```python
from build123d import *

# Parameters (mm, degrees)
F1_DEPTH = 144
F2_W     = 86
F2_H     = 4
F2_W_2   = 4
F2_H_2   = 25
F3_DEPTH = 15
F4_W     = 54.916096
F4_H     = 4
F4_W_2   = 4
F4_H_2   = 25
F5_DEPTH = 15


with BuildPart() as f1:
    # F0 (on Front) → F1 (new body)
    with BuildSketch(Plane.XZ):
        with BuildLine():
            Line((0, 37), (0, 2))
            ThreePointArc((0, 2), (0.585786, 0.585786), (2, 0))
            Line((2, 0), (6, 0))
            ThreePointArc((6, 0), (7.414214, 0.585786), (8, 2))
            Line((8, 2), (8, 32.406905))
            Line((8, 32.406905), (20.7, 32.406905))
            Line((20.7, 32.406905), (20.7, 2))
            ThreePointArc((20.7, 2), (21.285786, 0.585786), (22.7, 0))
            Line((22.7, 0), (26.7, 0))
            ThreePointArc((26.7, 0), (28.114214, 0.585786), (28.7, 2))
            Line((28.7, 2), (28.7, 32.406905))
            Line((28.7, 32.406905), (98.7, 32.406905))
            Line((98.7, 32.406905), (98.7, 33.406905))
            Line((98.7, 33.406905), (97.45, 33.406905))
            Line((97.45, 33.406905), (97.45, 34.806905))
            Line((97.45, 34.806905), (106.75, 34.806905))
            Line((106.75, 34.806905), (106.75, 33.406905))
            Line((106.75, 33.406905), (105, 33.406905))
            Line((105, 33.406905), (105, 32.406905))
            Line((105, 32.406905), (115, 32.406905))
            Line((115, 32.406905), (120, 32.406905))
            Line((120, 32.406905), (120, 38))
            ThreePointArc((120, 38), (119.414214, 39.414214), (118, 40))
            Line((118, 40), (3, 40))
            ThreePointArc((3, 40), (0.87868, 39.12132), (0, 37))
        make_face()
        with BuildLine():
            Line((120, 24.406905), (120, 32.406905))
            Line((120, 32.406905), (115, 32.406905))
            Line((115, 32.406905), (115, 24.406905))
            ThreePointArc((115, 24.406905), (115.585786, 22.992692), (117, 22.406905))
            Line((117, 22.406905), (118, 22.406905))
            ThreePointArc((118, 22.406905), (119.414214, 22.992692), (120, 24.406905))
        make_face()
    extrude(amount=F1_DEPTH)

    # F2 (on face) → F3 (cut)
    with BuildSketch(Plane.XZ.offset(144)):
        with Locations((53, 36)):
            Rectangle(F2_W, F2_H)
        with Locations((4, 15.5)):
            Rectangle(F2_W_2, F2_H_2)
        with Locations((24.7, 15.5)):
            Rectangle(F2_W_2, F2_H_2)
    extrude(amount=-F3_DEPTH, mode=Mode.SUBTRACT)

    # F4 (on Front) → F5 (cut)
    with BuildSketch(Plane.XZ):
        with Locations((37.458048, 36)):
            Rectangle(F4_W, F4_H)
        with Locations((4, 15.5)):
            Rectangle(F4_W_2, F4_H_2)
        with Locations((24.7, 15.5)):
            Rectangle(F4_W_2, F4_H_2)
    extrude(amount=F5_DEPTH, mode=Mode.SUBTRACT)


solid = f1.part
```
Read the model definition and answer for the solid it produces. Units are mm, in the model's axes. A direction names the side the tool comes from. Give positions to 0.01 mm unless a question says otherwise; leave off trailing zeros. Write each loop counter-clockwise with the first axis right and the second up, starting at its lowest first coordinate (ties: lowest second). Pieces come first, ordered by that corner, then holes. Notation, with made-up numbers: (54.5, 31) -> (61.5, 31) arc R31 cw to (61.5, 65) -> close; hole circle Ø1 at (57, 10). An arc over 180 degrees is marked (long way). Answer in a Markdown table with one row per item.
1) Section D-D on x = 31 is taken. Give the vertices of the cut face in (y, z).
Results list:
| item | result |
|---|---|
| outline | (-144, 32.41) -> (0, 32.41) -> (0, 34) -> (-15, 34) -> (-15, 38) -> (0, 38) -> (0, 40) -> (-144, 40) -> (-144, 38) -> (-129, 38) -> (-129, 34) -> (-144, 34) -> close |
2) Section A-A on z = 30 is taken. Give the vertices of the cut face in (x, y), plus the area to 3 significant figures.
Results list:
| item | result |
|---|---|
| outline | (0, -144) -> (8, -144) -> (8, 0) -> (0, 0) -> close; (20.7, -144) -> (28.7, -144) -> (28.7, 0) -> (20.7, 0) -> close; (115, -144) -> (120, -144) -> (120, 0) -> (115, 0) -> close |
| area | 3,020 mm^2 |
3) Section B-B on y = -93.5 is taken. Give the vertices of the cut face in (x, z).
Results list:
| item | result |
|---|---|
| outline | (0, 2) arc R2 ccw to (2, 0) -> (6, 0) arc R2 ccw to (8, 2) -> (8, 32.41) -> (20.7, 32.41) -> (20.7, 2) arc R2 ccw to (22.7, 0) -> (26.7, 0) arc R2 ccw to (28.7, 2) -> (28.7, 32.41) -> (98.7, 32.41) -> (98.7, 33.41) -> (97.45, 33.41) -> (97.45, 34.81) -> (106.75, 34.81) -> (106.75, 33.41) -> (105, 33.41) -> (105, 32.41) -> (115, 32.41) -> (115, 24.41) arc R2 ccw to (117, 22.41) -> (118, 22.41) arc R2 ccw to (120, 24.41) -> (120, 38) arc R2 ccw to (118, 40) -> (3, 40) arc R3 ccw to (0, 37) -> close |
4) A tool of negligible diameter and unlimited length cuts with its end or side. For faces 4 (the cylindrical face through (0.9, -70.99, 39.14)), 5 (the flat face through (25, -7, 3)), 6 (the flat face through (2, -137, 15)), 7 (the flat face through (120, -71, 31)), 8 (the flat face through (110, -71, 32.407)), from which of +Z, -Z, +X, -X, +Y, -Y can it reach the whole face along a straight path? Write none if from no direction.
Results list:
| item | result |
|---|---|
| face 4 | +Z, -X, +Y, -Y |
| face 5 | +Y |
| face 6 | -Y |
| face 7 | +Z, -Z, +X, +Y, -Y |
| face 8 | -Z, +Y, -Y |
5) Section C-C on z = 18 is taken. Give the vertices of the cut face in (x, y).
Results list:
| item | result |
|---|---|
| outline | (0, -144) -> (2, -144) -> (2, -129) -> (6, -129) -> (6, -144) -> (8, -144) -> (8, 0) -> (6, 0) -> (6, -15) -> (2, -15) -> (2, 0) -> (0, 0) -> close; (20.7, -144) -> (22.7, -144) -> (22.7, -129) -> (26.7, -129) -> (26.7, -144) -> (28.7, -144) -> (28.7, 0) -> (26.7, 0) -> (26.7, -15) -> (22.7, -15) -> (22.7, 0) -> (20.7, 0) -> close |
6) Each of these flat-tipped pins is pushed along its axis until it touches: pin 1 Ø2 at (x, y) = (106, -25.5) entering from -Z; pin 2 Ø4 at (y, z) = (-101, 9.5) entering from +X; pin 3 Ø7.5 at (y, z) = (-10, 20.5) entering from +X. Where does it stop, or does it pass through?
Results list:
| item | result |
|---|---|
| pin 1 | z = 32.41 |
| pin 2 | x = 28.7 |
| pin 3 | x = 119.99 |
7) Straight lines are drawn through the part: line 1 (X direction, y = -87, z = 28.5); line 2 (X direction, y = -11, z = 11.5); line 3 (Z direction, x = 61, y = -132). For each, find the intervals that lie inside material, in ascending order. Write a range as [from, to].
Results list:
| item | result |
|---|---|
| line 1 | [0, 8], [20.7, 28.7], [115, 120] |
| line 2 | [0, 2], [6, 8], [20.7, 22.7], [26.7, 28.7] |
| line 3 | [32.41, 34], [38, 40] |
8) Determine the mould class of faces 1 (the flat face through (52, -129, 36)), 2 (the flat face through (115, -71, 28)), 3 (the flat face through (63, -71, 32.407)) for opening direction Z: released by +Z, released by -Z, zero draft, split by the parting line, or undercut.
Results list:
| item | result |
|---|---|
| face 1 | undercut |
| face 2 | zero draft |
| face 3 | released by -Z |
